Work out the finished part from the listing and answer in its coordinate system (mm). A direction names the side the tool comes from. Give positions to 0.01 mm unless a question says otherwise; leave off trailing zeros. Order: outer loops, then holes, each group sorted by start corner. A loop starts at its lowest first (then second) coordinate and runs counter-clockwise, first axis right, second up. Notation, with made-up numbers: M 65.5,21 L 102.5,21 A15 cw 102.5,31 Z; hole C 68.5,-35.75 d10. An arc over 180 degrees is marked long. One line per item, written item: value.
from build123d import *

# Parameters (mm, degrees)
F0_W     = 76.2
F0_H     = 1219.2
F1_DEPTH = 38.1
F2_W     = 76.2
F2_H     = 38.1
F3_DEPTH = 2438.4
F4_START = 2476.5
F4_DEPTH = 38.1


with BuildPart() as f1:
    # F0 (on Top) → F1 (new body)
    with BuildSketch(Plane.XY):
        with Locations((-79.2764335848, -16.3942715153)):
            Rectangle(F0_W, F0_H)
    extrude(amount=F1_DEPTH)

    # F2 (on face) → F3 (join)
    with BuildSketch(Plane.XY.offset(38.1)):
        with Locations((-79.2764335848, -606.9442715153)):
            Rectangle(F2_W, F2_H)
        with Locations((-79.2764335848, 574.1557284847)):
            Rectangle(F2_W, F2_H)
        with Locations((-79.2764335848, 180.4557284847)):
            Rectangle(F2_W, F2_H)
        with Locations((-79.2764335848, -213.2442715153)):
            Rectangle(F2_W, F2_H)
    extrude(amount=F3_DEPTH)

    # F0 (on Top) → F4 (join)
    with BuildSketch(Plane.XY.offset(F4_START)):
        with Locations((-79.2764335848, -16.3942715153)):
            Rectangle(F0_W, F0_H)
    extrude(amount=F4_DEPTH)


solid = f1.part
(1) Find the intervals of material crossed by probe 1 along Y at (x, z) = (-73, 2245); probe 2 along Z at (x, y) = (-74, 478.5), in increasing order. Write a range as from..to.
Findings:
probe 1: y = -625.99..-587.89, -232.29..-194.19, 161.41..199.51, 555.11..593.21
probe 2: z = 0..38.1, 2476.5..2514.6
(2) Section B-B, the plane y = -486 is taken. Give the vertices of the cut face in (x, z).
Findings:
outline: M -117.38,0 L -41.18,0 L -41.18,38.1 L -117.38,38.1 Z; M -117.38,2476.5 L -41.18,2476.5 L -41.18,2514.6 L -117.38,2514.6 Z
(3) Determine the mould class of faces 1 (the flat face through (-80, -625.994, 1240)), 2 (the flat face through (-80, -587.894, 1240)), 3 (the flat face through (-117.376, -200, 1251)), 4 (the flat face through (-80, 380, 2476.5)) for opening direction Y: pulls with the +Y half, pulls with the -Y half, needs draft (parallel to the pull), parting line crosses it, or undercut.
Findings:
face 1: pulls with the -Y half
face 2: undercut
face 3: needs draft
face 4: undercut
(4) Which of the six approach directions +Z, -Z, +X, -X, +Y, -Y give full straight-line access (tool end or side, diameter ignored) to faces 5 (the flat face through (-80, -408, 38.1)), 6 (the flat face through (-80, -8, 0))?
Findings:
face 5: +X, -X
face 6: -Z, +X, -X, +Y, -Y
(5) Section A-A, the plane z = 1473.5 is taken. Give the vertices of the cut face in (x, y), then the cut area to 3 significant figures.
Findings:
outline: M -117.38,-625.99 L -41.18,-625.99 L -41.18,-587.89 L -117.38,-587.89 Z; M -117.38,-232.29 L -41.18,-232.29 L -41.18,-194.19 L -117.38,-194.19 Z; M -117.38,161.41 L -41.18,161.41 L -41.18,199.51 L -117.38,199.51 Z; M -117.38,555.11 L -41.18,555.11 L -41.18,593.21 L -117.38,593.21 Z
area: 11,600 mm^2
(6) Section C-C, the plane x = -75.5 is taken. Give the vertices of the cut face in (y, z), then the cut area to 3 significant figures.
Findings:
outline: M -625.99,0 L 593.21,0 L 593.21,2514.6 L -625.99,2514.6 Z; hole M -587.89,38.1 L -232.29,38.1 L -232.29,2476.5 L -587.89,2476.5 Z; hole M -194.19,38.1 L 161.41,38.1 L 161.41,2476.5 L -194.19,2476.5 Z; hole M 199.51,38.1 L 555.11,38.1 L 555.11,2476.5 L 199.51,2476.5 Z
area: 465,000 mm^2
